Part model, mm, in its own coordinate system. Face numbers are marked on the shaded views. A direction names the side the tool comes from. Give positions to 0.01 mm unless a question says otherwise; leave off trailing zeros. Order: outer loops, then holes, each group sorted by start corner. A loop starts at its lowest first (then second) coordinate and runs counter-clockwise, first axis right, second up.
1. Mould opens along Y. For the marked faces 1, 2 and 3 say: +Y half, -Y half, draft (parallel to the pull), parting line (faces both ways), or undercut.
2. Drop flat-ended pins along their axis: pin 1 Ø4.5 at (x, y) = (-46.5, 8.5) entering from +Z; pin 2 Ø5 at (x, y) = (39, -10) entering from +Z; pin 3 Ø1 at (x, y) = (22, 0) entering from +Z. Give the stop position or say it passes through.
3. Slice it at D-D on z = -3. List the corners of the cut face in (x, y), and give its area (3 significant figures).
4. Probe line 1 (Y direction, x = -18.5, z = -7); line 2 (Z direction, x = 14.5, y = 1.5); line 3 (Z direction, x = -45, y = 5.75). List the from-to ranges inside material, lowest first.
5. Which spindle directions (+Z, -Z, +X, -X, +Y, -Y) get a long thin tool onto all of the face, cutting with end or side? Do the marked faces 4, 5, 6 and 7. Say none if no direction does.
6. Slice it at B-B on x = 11.5. List the corners of the cut face in (y, z).
7. Slice it at A-A on z = -19.5. List the corners of the cut face in (x, y).
8. Slice it at C-C on y = 3. List the corners of the cut face in (x, z).
Solid Edge part; units mm, degrees
sketch "Sketch1" plane through (0, 0, 0) normal (0, 0, 1) x (1, 0, 0)
  line L0 (-60.5, -14) -> (60.5, -14)
  line L1 (60.5, -14) -> (60.5, 14)
  line L2 (60.5, 14) -> (-60.5, 14)
  line L3 (-60.5, 14) -> (-60.5, -14)
extrude "Protrusion1" add sketch "Sketch1" against normal blind 40
sketch "Sketch2" plane through (0, -14, -20) normal (0, -1, 0) x (1, 0, 0)
  line L0 (60.5, 20) -> (42, 20)
  line L1 (42, 20) -> (42, 11.5)
  line L2 (42, 11.5) -> (60.5, 11.5)
  line L3 (60.5, 11.5) -> (60.5, 20)
extrude "ExtrudedCutout_11" cut sketch "Sketch2" against normal blind 28
sketch "Sketch3" plane through (0, -14, -20) normal (0, -1, 0) x (1, 0, 0)
  line L0 (-60.5, 11.5) -> (-42, 11.5)
  line L1 (-42, 11.5) -> (-42, 20)
  line L2 (-42, 20) -> (-60.5, 20)
  line L3 (-60.5, 20) -> (-60.5, 11.5)
extrude "ExtrudedCutout_12" cut sketch "Sketch3" against normal blind 28
chamfer "Chamfer_7" [suppressed]
chamfer "Chamfer_8" [suppressed]
sketch "Sketch4" plane through (0, 0, 0) normal (0, 0, 1) x (0, 1, 0)
  line L0 (-4.9, -60.5) -> (4.9, -60.5)
  line L1 (4.9, -60.5) -> (4.9, 60.5)
  line L2 (4.9, 60.5) -> (-4.9, 60.5)
  line L3 (-4.9, 60.5) -> (-4.9, -60.5)
extrude "ExtrudedCutout_28" cut sketch "Sketch4" against normal blind 33
chamfer "Chamfer_9" distance 18 distance2 2.7 1 edges at (-60.5, 0, -33) measured on face at (-41.5433, -3.1687, -33)
chamfer "Chamfer_10" distance 18 distance2 2.7 1 edges at (-60.5, -4.9, -22.1) measured on face at (-41.5433, -4.9, -29.393)
chamfer "Chamfer_11" distance 18 distance2 2.7 1 edges at (-60.5, 4.9, -22.1) measured on face at (41.5433, 4.9, -29.393)
chamfer "Chamfer_12" distance 18 distance2 2.7 1 edges at (60.5, 0, -33) measured on face at (-26.3633, -3.1687, -33)
chamfer "Chamfer_13" distance 18 distance2 2.7 1 edges at (60.5, 4.9, -22.1) measured on face at (44.3633, 4.9, -29.393)
chamfer "Chamfer_14" distance 18 distance2 2.7 1 edges at (60.5, -4.9, -22.1) measured on face at (-26.3633, -4.9, -29.393)
sketch "Sketch5" plane through (0, -14, -20) normal (0, -1, 0) x (1, 0, 0)
  line L0 (-36, 20) -> (-42, 11.5)
  line L1 (-42, 11.5) -> (-42, 20)
  line L2 (-42, 20) -> (-36, 20)
  line L3 (36, 20) -> (42, 11.5)
  line L4 (42, 11.5) -> (42, 20)
  line L5 (42, 20) -> (36, 20)
extrude "ExtrudedCutout_29" cut sketch "Sketch5" against normal blind 30
chamfer "Chamfer_15" distance 3.8 angle 45 4 edges at (60.5, 10.8, -8.5) (60.5, -10.8, -8.5) (-60.5, 10.8, -8.5) (-60.5, -10.8, -8.5)
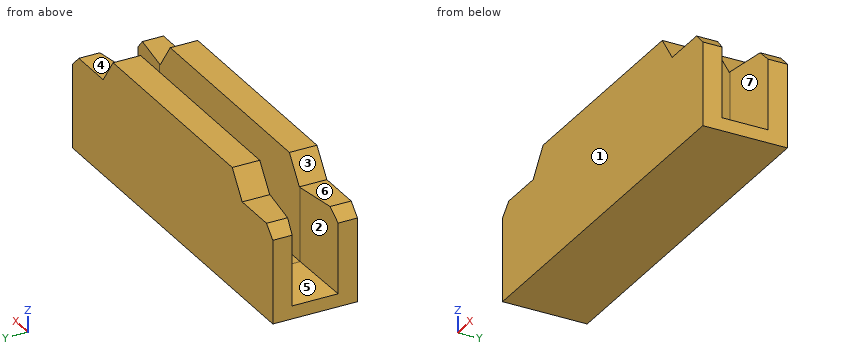
Data:
1. face 1: -Y half
1. face 2: undercut
1. face 3: draft
2. pin 1: stops at z = -8.5
2. pin 2: stops at z = -0.71
2. pin 3: stops at z = -33
3. outline: (-38.12, -14) - (38.12, -14) - (38.12, -4.9) - (-38.12, -4.9) - close; (-38.12, 4.9) - (38.12, 4.9) - (38.12, 14) - (-38.12, 14) - close
3. area: 1,390 mm2
4. line 1: y = -14 to -4.9, 4.9 to 14
4. line 2: z = -40 to -33
4. line 3: z = -40 to -8.5
5. face 4: +Z, +X, +Y, -Y
5. face 5: +Z, -X
5. face 6: +Z, -X, +Y, -Y
5. face 7: +Z, +X
6. outline: (-14, -40) - (14, -40) - (14, 0) - (4.9, 0) - (4.9, -33) - (-4.9, -33) - (-4.9, 0) - (-14, 0) - close
7. outline: (-60.5, -14) - (60.5, -14) - (60.5, -7.6) - (42.5, -4.9) - (-42.5, -4.9) - (-60.5, -7.6) - close; (-60.5, 7.6) - (-42.5, 4.9) - (42.5, 4.9) - (60.5, 7.6) - (60.5, 14) - (-60.5, 14) - close
8. outline: (-60.5, -40) - (60.5, -40) - (60.5, -35.7) - (42.5, -33) - (-42.5, -33) - (-60.5, -35.7) - close
